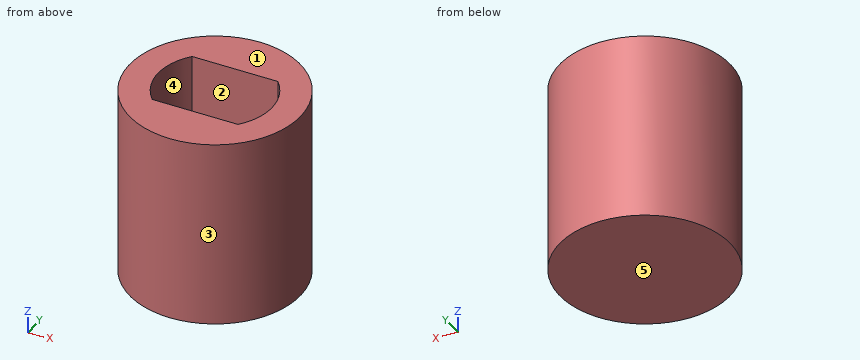
```python
from build123d import *

# Parameters (mm, degrees)
EXTRUDE001_DEPTH = 7
CYLINDER_R       = 4.5
CYLINDER_DEPTH   = 10


with BuildPart() as extrude001:
    # Sketch002 (on Face3 of Cylinder) → Extrude001 (new body)
    with BuildSketch(Plane.XY.offset(10)):
        with BuildLine():
            ThreePointArc((2.236068, -2), (3, 0), (2.236068, 2))
            Line((-2.236068, 2), (2.236068, 2))
            ThreePointArc((-2.236068, 2), (-3, 0), (-2.236068, -2))
            Line((2.236068, -2), (-2.236068, -2))
        make_face()
    extrude(amount=-EXTRUDE001_DEPTH)


with BuildPart() as cut_for_support:
    # Cylinder → Cylinder (new body)
    with BuildSketch(Plane.XY):
        Circle(CYLINDER_R)
    extrude(amount=CYLINDER_DEPTH)

    # Cut001: cut Extrude001
    add(extrude001.part, mode=Mode.SUBTRACT)


solid = cut_for_support.part
```
Model file for the job. Use its own axes, mm. Face numbers are marked on the shaded views. A direction names the side the tool comes from. Give positions to 0.01 mm unless a question says otherwise; leave off trailing zeros. Loops run counter-clockwise (first coordinate to the right, second up) from the corner with the lowest first, then second, coordinate; pieces in that order, holes last. Notation, with made-up numbers: (-21, -31.5) -> (18, -31.5) arc R17 cw to (18, -16.5) -> close; hole circle Ø5 at (85.5, -38). An arc over 180 degrees is marked (long way). Write each question's results on one line, items separated by ' | '.
(1) Probe line 1 along Y through (x, z) = (0, 5); line 2 along Z through (x, y) = (1.25, 1); line 3 along Y through (x, z) = (-2, 7). List the from-to ranges inside material, lowest first.
Geometry results:
line 1: y = -4.5 to -2, 2 to 4.5 | line 2: z = 0 to 3 | line 3: y = -4.03 to -2, 2 to 4.03
(2) Cut at D-D on z = 1. List the corners of the cut face in (x, y), and give its area (3 significant figures).
Geometry results:
outline: circle Ø9 at (0, 0) | area: 63.6 mm²
(3) Flat gauge pin, fed straight in: pin 1 Ø1.5 at (x, z) = (1, 4) entering from +Y. Where does the tip first touch, or does it go through?
Geometry results:
pin 1: stops at y = 4.49
(4) Pull direction X, two halves, no side cores. Call the marked faces 3, 4 and 5: released by +X, released by -X, zero draft, split by the parting line, or undercut.
Geometry results:
face 3: split by the parting line | face 4: undercut | face 5: zero draft
(5) Tool access for the marked faces 1 and 2: list every direction of +Z, -Z, +X, -X, +Y, -Y with a clear straight run to the whole face (end or side of a thin tool).
Geometry results:
face 1: +Z, +X, -X, +Y, -Y | face 2: +Z
(6) Cut at B-B on z = 6.5. List the corners of the cut face in (x, y), and give its area (3 significant figures).
Geometry results:
outline: circle Ø9 at (0, 0); hole (-2.24, -2) -> (2.24, -2) arc R3 ccw to (2.24, 2) -> (-2.24, 2) arc R3 ccw to start | area: 41.5 mm²
(7) Cut at A-A on x = 0. List the corners of the cut face in (y, z).
Geometry results:
outline: (-4.5, 0) -> (4.5, 0) -> (4.5, 10) -> (2, 10) -> (2, 3) -> (-2, 3) -> (-2, 10) -> (-4.5, 10) -> close
(8) Cut at C-C on y = 0. List the corners of the cut face in (x, z).
Geometry results:
outline: (-4.5, 0) -> (4.5, 0) -> (4.5, 10) -> (3, 10) -> (3, 3) -> (-3, 3) -> (-3, 10) -> (-4.5, 10) -> close
